```python
from build123d import *

# Parameters (mm, degrees)
SKETCH5_W           = 10.2
SKETCH5_H           = 6.78
SKETCH16_W          = 7.3
SKETCH16_H          = 8.75
CUT_TOOTH_START     = -10.2
CUT_TOOTH_DEPTH     = 10.2
PATTERN_TOOTH_COUNT = 15
SKETCH_1_R          = 2.5
CUT_EXTRUDE_1_DEPTH = 20
SKETCH_2_R          = 1
CUT_EXTRUDE_2_DEPTH = 10


with BuildPart() as part:
    # Sketch5 → body (revolve)
    with BuildSketch(Plane(origin=(0, 0, 0), x_dir=(0, 0, -1), z_dir=(1, 0, 0)), mode=Mode.PRIVATE) as body_sk:
        with Locations((5.1, 3.39)):
            Rectangle(SKETCH5_W, SKETCH5_H)
    revolve(body_sk.sketch.rotate(Axis((0, 0, 0), (0, 0, -1)), 90), axis=Axis((0, 0, 0), (0, 0, -1)))

    # Sketch16 → body-hub (revolve)
    with BuildSketch(Plane(origin=(0, 0, 0), x_dir=(0, 0, -1), z_dir=(1, 0, 0)), mode=Mode.PRIVATE) as body_hub_sk:
        with Locations((13.85, 4.375)):
            Rectangle(SKETCH16_W, SKETCH16_H)
    revolve(body_hub_sk.sketch.rotate(Axis((0, 0, -17.5), (0, 0, 1)), 90), axis=Axis((0, 0, -17.5), (0, 0, 1)))

    # Sketch23 → cut-tooth (cut)
    with BuildSketch(Plane.XY.offset(CUT_TOOTH_START)):
        with BuildLine():
            Line((0.7, 6.28), (0.7, 6.518159249))
            ThreePointArc((0.7, 6.518159249), (0.768605793, 6.668942413), (0.927355623, 6.716279591))
            Line((0.927355623, 6.716279591), (0.927355623, 7.852559183))
            Line((0.927355623, 7.852559183), (-0.927355623, 7.852559183))
            Line((-0.927355623, 7.852559183), (-0.927355623, 6.716279591))
            ThreePointArc((-0.927355623, 6.716279591), (-0.768605793, 6.668942413), (-0.7, 6.518159249))
            Line((-0.7, 6.518159249), (-0.7, 6.28))
            ThreePointArc((-0.7, 6.28), (0, 5.58), (0.7, 6.28))
        make_face()
    cut_tooth = extrude(amount=CUT_TOOTH_DEPTH, mode=Mode.SUBTRACT)

    # pattern-tooth: cut-tooth ×15 about axis
    pattern_tooth_axis = Axis((0, 0, -10.2), (0, 0, 1))
    for i in range(1, PATTERN_TOOTH_COUNT):
        add(cut_tooth.rotate(pattern_tooth_axis, i * 360 / PATTERN_TOOTH_COUNT), mode=Mode.SUBTRACT)

    # Sketch25 → body-flange-front (revolve)
    with BuildSketch(Plane(origin=(0, 0, 0), x_dir=(0, 0, -1), z_dir=(1, 0, 0)), mode=Mode.PRIVATE) as body_flange_front_sk:
        Polygon((0.5, 3.392), (0, 3.392), (0, 6.964), (0, 8.75), (0.5, 8.75), (0.5, 6.964), align=None)
    revolve(body_flange_front_sk.sketch.rotate(Axis((0, 0, 0), (0, 0, -1)), 90), axis=Axis((0, 0, 0), (0, 0, -1)))

    # Sketch28 → body-flange-profile-front (revolve, cut)
    with BuildSketch(Plane(origin=(0, 0, 0), x_dir=(0, 0, -1), z_dir=(1, 0, 0)), mode=Mode.PRIVATE) as body_flange_profile_front_sk:
        Polygon((0.5, 8.75), (0.5, 8.25), (0.266846171, 8.75), align=None)
    revolve(body_flange_profile_front_sk.sketch.rotate(Axis((0, 0, -10.2), (0, 0, 1)), 90), axis=Axis((0, 0, -10.2), (0, 0, 1)), mode=Mode.SUBTRACT)

    # 草图1 → 切除-拉伸1 (cut)
    with BuildSketch(Plane(origin=(0, 0, -17.5), x_dir=(-1, 0, 0), z_dir=(0, 0, -1))):
        Circle(SKETCH_1_R)
    extrude(amount=-CUT_EXTRUDE_1_DEPTH, mode=Mode.SUBTRACT)

    # 草图2 → 切除-拉伸2 (cut)
    with BuildSketch(Plane(origin=(0, 0, 0), x_dir=(1, 0, 0), z_dir=(0, 1, 0))):
        with Locations(Location((0, 14, 0), (0, 0, 270))):
            Circle(SKETCH_2_R)
    extrude(amount=-CUT_EXTRUDE_2_DEPTH, mode=Mode.SUBTRACT)


solid = part.part
```
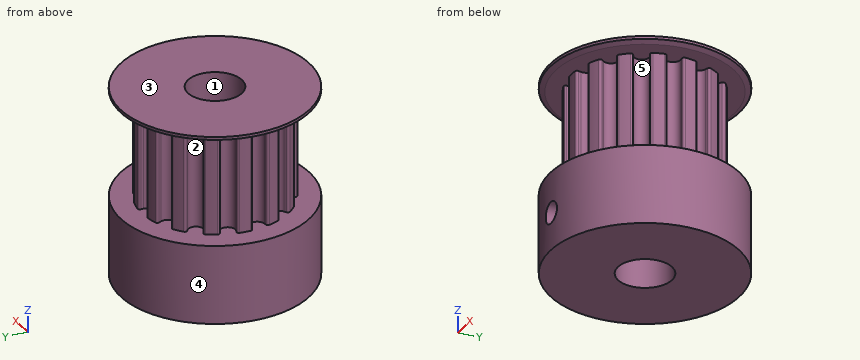
Model file for the job. Use its own axes, mm. Face numbers are marked on the shaded views. A direction names the side the tool comes from. Give positions to 0.01 mm unless a question says otherwise; leave off trailing zeros. Order: outer loops, then holes, each group sorted by start corner. A loop starts at its lowest first (then second) coordinate and runs counter-clockwise, first axis right, second up.
1) Saw through at A-A, the plane x = 0. Write the cut outline in (y, z), then the cut area to 3 significant figures.
2) Pin check, flat tips, straight feed: pin 1 (8 mm diameter, centred on x = 1, y = 0, fed in from -Z); pin 2 (1 mm diameter, centred on y = 7, z = -13.5, fed in from +X). Stop position of each tip, or through.
3) Saw through at B-B, the plane z = -14. Write the cut outline in (x, y), then the cut area to 3 significant figures.
4) Wall check: probe 1 along Z at (x, y) = (3, -6.5); probe 2 along Z at (x, y) = (0, -4.5); probe 3 along Y at (x, z) = (0, -8.5). Give the ranges that are in metal, low to high.
5) 3-axis set-ups, long thin cutter, end or side, ignore diameter. For the marked faces 1 and 2: which of +Z, -Z, +X, -X, +Y, -Y reach the whole face in a straight line?
6) Mould opens along Y. For the marked faces 3, 4 and 5 say: +Y half, -Y half, draft (parallel to the pull), parting line (faces both ways), or undercut.
Computed:
1. outline: (-8.75, -17.5) - (-2.5, -17.5) - (-2.5, -15) - (-8.75, -15) - close; (-8.75, -13) - (-2.5, -13) - (-2.5, 0) - (-8.75, 0) - (-8.75, -0.27) - (-8.25, -0.5) - (-6.78, -0.5) - (-6.78, -10.2) - (-8.75, -10.2) - close; (2.5, -17.5) - (8.75, -17.5) - (8.75, -10.2) - (5.58, -10.2) - (5.58, -0.5) - (8.25, -0.5) - (8.75, -0.27) - (8.75, 0) - (2.5, 0) - close
1. area: 156 mm2
2. pin 1: stops at z = -17.5
2. pin 2: stops at x = 5.86
3. outline: (-1, -8.69) - (-1, -2.29) arc R2.5 cw (long way) to (1, -2.29) - (1, -8.69) arc R8.75 ccw (long way) to start
3. area: 208 mm2
4. probe 1: z = -17.5 to -10.2, -0.5 to 0
4. probe 2: z = -17.5 to -15, -13 to 0
4. probe 3: y = -6.78 to -2.5, 2.5 to 5.58
5. face 1: +Z, -Z
5. face 2: none
6. face 3: draft
6. face 4: parting line
6. face 5: undercut
